from build123d import *
from OCP.BRepFilletAPI import BRepFilletAPI_MakeChamfer

# Parameters (mm, degrees)
SKETCH1_W           = 48
SKETCH1_H           = 65
BOSS_EXTRUDE1_DEPTH = 30
FILLET2_R           = 3
SKETCH2_R           = 9
BOSS_EXTRUDE2_DEPTH = 1
BOSS_EXTRUDE4_START = 1
SKETCH4_R           = 9
BOSS_EXTRUDE4_DEPTH = 1
SKETCH5_R           = 3
BOSS_EXTRUDE5_DEPTH = 6
CHAMFER1_SIZE       = 3
CHAMFER1_SIZE2      = 1.000002977
CHAMFER2_SIZE       = 1
CHAMFER3_SIZE       = 2.5
CHAMFER3_SIZE2      = 0.99992866
SKETCH6_R           = 3
SKETCH6_R_2         = 2.5
BOSS_EXTRUDE6_DEPTH = 2.5
SKETCH7_R           = 2.500002977
SKETCH7_R_2         = 3
BOSS_EXTRUDE7_DEPTH = 3
SKETCH8_R           = 1.25
CUT_EXTRUDE1_DEPTH  = 5
SKETCH10_R          = 1.25
CUT_EXTRUDE2_DEPTH  = 5


with BuildPart() as part:
    # Sketch1 → Boss-Extrude1 (new body)
    with BuildSketch(Plane(origin=(0, 0, 0), x_dir=(1, 0, 0), z_dir=(0, 1, 0))):
        Rectangle(SKETCH1_W, SKETCH1_H)
    extrude(amount=BOSS_EXTRUDE1_DEPTH)

    # Fillet2
    fillet2_edges = [part.edges().sort_by_distance(p)[0] for p in [
        (0, 30, -32.5),
        (0, 0, -32.5),
        (0, 0, 32.5),
        (0, 30, 32.5),
    ]]
    fillet(fillet2_edges, radius=FILLET2_R)

    # Sketch2 → Boss-Extrude2 (add)
    with BuildSketch(Plane.ZY.offset(24)):
        with Locations(Location((19.5, 15, 0), (0, 0, 180))):
            Circle(SKETCH2_R)
    extrude(amount=BOSS_EXTRUDE2_DEPTH)

    # Sketch4 → Boss-Extrude4 (add)
    with BuildSketch(Plane(origin=(24, 0, 0), x_dir=(0, 0, -1), z_dir=(1, 0, 0)).offset(BOSS_EXTRUDE4_START)):
        with Locations((-19.5, 15)):
            Circle(SKETCH4_R)
    extrude(amount=-BOSS_EXTRUDE4_DEPTH)

    # Sketch5 → Boss-Extrude5 (add)
    with BuildSketch(Plane(origin=(25, 0, 0), x_dir=(0, 0, -1), z_dir=(1, 0, 0))):
        with Locations((-19.5, 15)):
            Circle(SKETCH5_R)
    extrude(amount=BOSS_EXTRUDE5_DEPTH)

    # Chamfer1: one chamfer whose edges measure the first distance from different faces: ONE call of the kernel's chamfer builder (chamfer() names one face for all edges)
    chamfer1_edges_1 = [part.edges().sort_by_distance(p)[0] for p in [
        (-24, 30, 0),
    ]]
    chamfer1_side_1 = [part.faces().sort_by_distance(p)[0] for p in [
        (0, 30, 0),
    ]]
    chamfer1_edges_2 = [part.edges().sort_by_distance(p)[0] for p in [
        (-24, 0, 0),
    ]]
    chamfer1_side_2 = [part.faces().sort_by_distance(p)[0] for p in [
        (0, 0, 0),
    ]]
    chamfer1_edges_3 = [part.edges().sort_by_distance(p)[0] for p in [
        (-24, 15, 32.5),
    ]]
    chamfer1_side_3 = [part.faces().sort_by_distance(p)[0] for p in [
        (0, 15, 32.5),
    ]]
    chamfer1_edges_4 = [part.edges().sort_by_distance(p)[0] for p in [
        (-24, 15, -32.5),
    ]]
    chamfer1_side_4 = [part.faces().sort_by_distance(p)[0] for p in [
        (0, 15, -32.5),
    ]]
    chamfer1_edges_5 = [part.edges().sort_by_distance(p)[0] for p in [
        (-24, 29.121320344, 31.621320344),
    ]]
    chamfer1_side_5 = [part.faces().sort_by_distance(p)[0] for p in [
        (0, 29.121320344, 31.621320344),
    ]]
    chamfer1_edges_6 = [part.edges().sort_by_distance(p)[0] for p in [
        (-24, 0.878679656, 31.621320344),
    ]]
    chamfer1_side_6 = [part.faces().sort_by_distance(p)[0] for p in [
        (0, 0.878679656, 31.621320344),
    ]]
    chamfer1_edges_7 = [part.edges().sort_by_distance(p)[0] for p in [
        (-24, 0.878679656, -31.621320344),
    ]]
    chamfer1_side_7 = [part.faces().sort_by_distance(p)[0] for p in [
        (0, 0.878679656, -31.621320344),
    ]]
    chamfer1_edges_8 = [part.edges().sort_by_distance(p)[0] for p in [
        (-24, 29.121320344, -31.621320344),
    ]]
    chamfer1_side_8 = [part.faces().sort_by_distance(p)[0] for p in [
        (0, 29.121320344, -31.621320344),
    ]]
    chamfer1 = BRepFilletAPI_MakeChamfer(part.part.solid().wrapped)
    for e in chamfer1_edges_1:
        chamfer1.Add(CHAMFER1_SIZE, CHAMFER1_SIZE2, e.wrapped, chamfer1_side_1[0].wrapped)  # the first distance lies on this face
    for e in chamfer1_edges_2:
        chamfer1.Add(CHAMFER1_SIZE, CHAMFER1_SIZE2, e.wrapped, chamfer1_side_2[0].wrapped)  # the first distance lies on this face
    for e in chamfer1_edges_3:
        chamfer1.Add(CHAMFER1_SIZE, CHAMFER1_SIZE2, e.wrapped, chamfer1_side_3[0].wrapped)  # the first distance lies on this face
    for e in chamfer1_edges_4:
        chamfer1.Add(CHAMFER1_SIZE, CHAMFER1_SIZE2, e.wrapped, chamfer1_side_4[0].wrapped)  # the first distance lies on this face
    for e in chamfer1_edges_5:
        chamfer1.Add(CHAMFER1_SIZE, CHAMFER1_SIZE2, e.wrapped, chamfer1_side_5[0].wrapped)  # the first distance lies on this face
    for e in chamfer1_edges_6:
        chamfer1.Add(CHAMFER1_SIZE, CHAMFER1_SIZE2, e.wrapped, chamfer1_side_6[0].wrapped)  # the first distance lies on this face
    for e in chamfer1_edges_7:
        chamfer1.Add(CHAMFER1_SIZE, CHAMFER1_SIZE2, e.wrapped, chamfer1_side_7[0].wrapped)  # the first distance lies on this face
    for e in chamfer1_edges_8:
        chamfer1.Add(CHAMFER1_SIZE, CHAMFER1_SIZE2, e.wrapped, chamfer1_side_8[0].wrapped)  # the first distance lies on this face
    add(Compound.cast(chamfer1.Shape()), mode=Mode.REPLACE)

    # Chamfer2
    chamfer2_edges = [part.edges().sort_by_distance(p)[0] for p in [
        (-25, 15, 28.5),
    ]]
    chamfer(chamfer2_edges, length=CHAMFER2_SIZE - 0.0001)  # a hair under: the kernel refuses the full size

    # Chamfer3: one chamfer whose edges measure the first distance from different faces: ONE call of the kernel's chamfer builder (chamfer() names one face for all edges)
    chamfer3_edges_1 = [part.edges().sort_by_distance(p)[0] for p in [
        (24, 30, 0),
    ]]
    chamfer3_side_1 = [part.faces().sort_by_distance(p)[0] for p in [
        (1.5, 30, 0),
    ]]
    chamfer3_edges_2 = [part.edges().sort_by_distance(p)[0] for p in [
        (24, 15, -32.5),
    ]]
    chamfer3_side_2 = [part.faces().sort_by_distance(p)[0] for p in [
        (1.5, 15, -32.5),
    ]]
    chamfer3_edges_3 = [part.edges().sort_by_distance(p)[0] for p in [
        (24, 0, 0),
    ]]
    chamfer3_side_3 = [part.faces().sort_by_distance(p)[0] for p in [
        (1.5, 0, 0),
    ]]
    chamfer3_edges_4 = [part.edges().sort_by_distance(p)[0] for p in [
        (24, 15, 32.5),
    ]]
    chamfer3_side_4 = [part.faces().sort_by_distance(p)[0] for p in [
        (1.5, 15, 32.5),
    ]]
    chamfer3_edges_5 = [part.edges().sort_by_distance(p)[0] for p in [
        (24, 29.121320344, 31.621320344),
    ]]
    chamfer3_side_5 = [part.faces().sort_by_distance(p)[0] for p in [
        (1.5, 29.121320344, 31.621320344),
    ]]
    chamfer3_edges_6 = [part.edges().sort_by_distance(p)[0] for p in [
        (24, 0.878679656, 31.621320344),
    ]]
    chamfer3_side_6 = [part.faces().sort_by_distance(p)[0] for p in [
        (1.5, 0.878679656, 31.621320344),
    ]]
    chamfer3_edges_7 = [part.edges().sort_by_distance(p)[0] for p in [
        (24, 0.878679656, -31.621320344),
    ]]
    chamfer3_side_7 = [part.faces().sort_by_distance(p)[0] for p in [
        (1.5, 0.878679656, -31.621320344),
    ]]
    chamfer3_edges_8 = [part.edges().sort_by_distance(p)[0] for p in [
        (24, 29.121320344, -31.621320344),
    ]]
    chamfer3_side_8 = [part.faces().sort_by_distance(p)[0] for p in [
        (1.5, 29.121320344, -31.621320344),
    ]]
    chamfer3 = BRepFilletAPI_MakeChamfer(part.part.solid().wrapped)
    for e in chamfer3_edges_1:
        chamfer3.Add(CHAMFER3_SIZE, CHAMFER3_SIZE2, e.wrapped, chamfer3_side_1[0].wrapped)  # the first distance lies on this face
    for e in chamfer3_edges_2:
        chamfer3.Add(CHAMFER3_SIZE, CHAMFER3_SIZE2, e.wrapped, chamfer3_side_2[0].wrapped)  # the first distance lies on this face
    for e in chamfer3_edges_3:
        chamfer3.Add(CHAMFER3_SIZE, CHAMFER3_SIZE2, e.wrapped, chamfer3_side_3[0].wrapped)  # the first distance lies on this face
    for e in chamfer3_edges_4:
        chamfer3.Add(CHAMFER3_SIZE, CHAMFER3_SIZE2, e.wrapped, chamfer3_side_4[0].wrapped)  # the first distance lies on this face
    for e in chamfer3_edges_5:
        chamfer3.Add(CHAMFER3_SIZE, CHAMFER3_SIZE2, e.wrapped, chamfer3_side_5[0].wrapped)  # the first distance lies on this face
    for e in chamfer3_edges_6:
        chamfer3.Add(CHAMFER3_SIZE, CHAMFER3_SIZE2, e.wrapped, chamfer3_side_6[0].wrapped)  # the first distance lies on this face
    for e in chamfer3_edges_7:
        chamfer3.Add(CHAMFER3_SIZE, CHAMFER3_SIZE2, e.wrapped, chamfer3_side_7[0].wrapped)  # the first distance lies on this face
    for e in chamfer3_edges_8:
        chamfer3.Add(CHAMFER3_SIZE, CHAMFER3_SIZE2, e.wrapped, chamfer3_side_8[0].wrapped)  # the first distance lies on this face
    add(Compound.cast(chamfer3.Shape()), mode=Mode.REPLACE)

    # Sketch6 → Boss-Extrude6 (add)
    with BuildSketch(Plane(origin=(24, 0, 0), x_dir=(0, 0, -1), z_dir=(1, 0, 0))):
        with Locations((6, 27)):
            Circle(SKETCH6_R)
        with Locations((6, 3)):
            Circle(SKETCH6_R)
        with Locations((-30, 3)):
            Circle(SKETCH6_R_2)
        with Locations((-30, 27)):
            Circle(SKETCH6_R_2)
        with Locations((30, 27)):
            Circle(SKETCH6_R_2)
        with Locations((30, 3)):
            Circle(SKETCH6_R_2)
    extrude(amount=-BOSS_EXTRUDE6_DEPTH)

    # Sketch7 → Boss-Extrude7 (add)
    with BuildSketch(Plane.ZY.offset(24)):
        with Locations((-29.999997023, 15)):
            Circle(SKETCH7_R)
        with Locations((-17.999997023, 3)):
            Circle(SKETCH7_R_2)
        with Locations((-17.999997023, 27)):
            Circle(SKETCH7_R_2)
    extrude(amount=-BOSS_EXTRUDE7_DEPTH)

    # Sketch8 → Cut-Extrude1 (cut)
    with BuildSketch(Plane.ZY.offset(24)):
        with Locations((-17.999997023, 27)):
            Circle(SKETCH8_R)
        with Locations((-29.999997023, 15)):
            Circle(SKETCH8_R)
        with Locations((-17.999997023, 3)):
            Circle(SKETCH8_R)
    extrude(amount=-CUT_EXTRUDE1_DEPTH, mode=Mode.SUBTRACT)

    # Sketch10 → Cut-Extrude2 (cut)
    with BuildSketch(Plane(origin=(24, 0, 0), x_dir=(0, 0, -1), z_dir=(1, 0, 0))):
        with Locations((6, 3)):
            Circle(SKETCH10_R)
        with Locations((30, 3)):
            Circle(SKETCH10_R)
        with Locations((6, 27)):
            Circle(SKETCH10_R)
        with Locations((30, 27)):
            Circle(SKETCH10_R)
        with Locations((-30, 3)):
            Circle(SKETCH10_R)
        with Locations((-30, 27)):
            Circle(SKETCH10_R)
    extrude(amount=-CUT_EXTRUDE2_DEPTH, mode=Mode.SUBTRACT)


solid = part.part
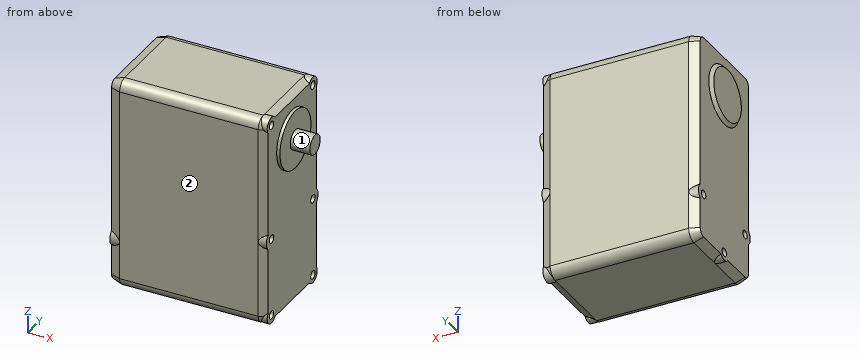
The listing builds one solid part. Answer for the finished solid, in the listing's coordinates (mm). Face numbers are marked on the shaded views. A direction names the side the tool comes from. Give positions to 0.01 mm unless a question says otherwise; leave off trailing zeros. Order: outer loops, then holes, each group sorted by start corner. A loop starts at its lowest first (then second) coordinate and runs counter-clockwise, first axis right, second up. Notation, with made-up numbers: (-25.75, 14) -> (11.25, 14) arc R9 cw to (11.25, 23) -> close; hole circle Ø1 at (-13, 14). An arc over 180 degrees is marked (long way). Put each result on its own line as item: value.
Item 1: Straight lines are drawn through the part: line 1 (Y direction, x = 23, z = -30); line 2 (X direction, y = 15, z = -27.5); line 3 (Y direction, x = 22, z = -30) (3 decimals). For each, find the intervals that lie inside material, in ascending order.
Established:
line 1: y = 0.5 to 1.75, 4.25 to 25.75, 28.25 to 29.5
line 2: x = -24 to 24
line 3: y = 0.245 to 1.75, 4.25 to 25.75, 28.25 to 29.755
Item 2: A cutting plane is placed at B-B on x = 26.5. Give the vertices of the cut face in (y, z), plus the area to 3 significant figures.
Established:
outline: circle Ø6 at (15, 19.5)
area: 28.3 mm^2
Item 3: For the marked faces 1 and 2, determine the directions among +Z, -Z, +X, -X, +Y, -Y from which every point of the face is accessible in a straight line to the end or side of a thin tool.
Established:
face 1: +X
face 2: +Z, -Z, +X, -X, -Y
Item 4: Given P1, Ø4, axis at y = 15, z = -30, coming from the +X side; P2, Ø2, axis at y = 8.5, z = -5, coming from the -X side; P3, Ø1.2, axis at y = 27.5, z = -18, coming from the -X side; P4, Ø6, axis at y = 16.5, z = 23, coming from the +X side, each flat-ended and moving along its own axis, determine where each tip first touches the part or whether it passes through.
Established:
P1: stops at x = 24
P2: stops at x = -24
P3: stops at x = -19
P4: stops at x = 31
